Check sheet for the modelled part. Datum: model origin and axes. Units: mm. A direction names the side the tool comes from. Give positions to 0.01 mm unless a question says otherwise; leave off trailing zeros. Loops run counter-clockwise (first coordinate to the right, second up) from the corner with the lowest first, then second, coordinate; pieces in that order, holes last. Notation, with made-up numbers: M 85.25,56 L 121.25,56 A18 ccw 121.25,90 Z; hole C 58.5,63 d11. An arc over 180 degrees is marked long. Write each question's results on one line, items separated by ' | '. Start each with the question number.
1. Sectioned sample at A-A on y = 0.75. Record the cut outline in (x, z), and give its area (3 significant figures).
2. Material ranges on line 1 along Z through (x, y) = (-1.5, 0.5); line 2 along X through (y, z) = (2.75, -0.75); line 3 along X through (y, z) = (1.75, -1.25), recorded low to high.
3. Draft check along X on faces 4 (the conical face through (-2.065, 4.936, -3.597)), 5 (the cylindrical face through (0.631, 4.892, -2.003)), 6 (the conical face through (2.083, 4.936, -3.587)). Enter one of: pulls with the +X half, pulls with the -X half, needs draft (parallel to the pull), parting line crosses it, or undercut.
4. Go/stop test with flat-tipped pins: pin 1 (2 mm diameter, centred on y = 3, z = 2.5, fed in from +X); pin 2 (4 mm diameter, centred on x = 0, z = 0, fed in from -Y); pin 3 (3 mm diameter, centred on y = 5.5, z = -2.5, fed in from +X); pin 4 (1 mm diameter, centred on y = 3.5, z = 3, fed in from -X). Record where each tip stops, or that it passes through.
5. Tool access check on faces 1 (the cylindrical face through (-0.1, 2, 2.5)), 2 (the conical face through (-4.15, 0.087, -0.01)), 3 (the cylindrical face through (3.905, 5.416, 0.867)). Record the directions out of +Z, -Z, +X, -X, +Y, -Y that give a thin tool (end or side, any length) a straight path to the whole face; none if there is none.
```python
from build123d import *

# Parameters (mm, degrees)
ESQUISSE2_OUTSIDE_W     = 16.754
ESQUISSE2_OUTSIDE_H     = 16.754
ENL_V_MAT_EXTRU_2_DEPTH = 7.3000001


with BuildPart() as part:
    # Esquisse1 → Base-Révolution (revolve)
    with BuildSketch(Plane.XY, mode=Mode.PRIVATE) as base_r_volution_sk:
        with BuildLine():
            Line((3, 5.800000004), (3.499999996, 5.800000004))
            Line((3.499999996, 5.800000004), (3.499999996, 4.33246532))
            Line((3.499999996, 4.33246532), (2.5, 4.064516129))
            Line((2.5, 4.064516129), (2.5, 0))
            Line((2.5, 0), (4, 0))
            Line((4, 0), (5.656854249, 0.956585264))
            Line((5.656854249, 0.956585264), (5.656854249, 4.064516129))
            Line((5.656854249, 4.064516129), (3.999999993, 5.02110138))
            Line((3.999999993, 5.02110138), (3.999999993, 5.800000004))
            ThreePointArc((3.999999993, 5.800000004), (3.499999996, 6.3), (3, 5.800000004))
        make_face()
    revolve(base_r_volution_sk.sketch.rotate(Axis((0, 0, 0), (0, 1, 0)), 90), axis=Axis((0, 0, 0), (0, 1, 0)))  # turned: the seam where the file's is

    # Esquisse2 outside → Enlèv. mat.-Extru.2 (cut, through all)
    with BuildSketch(Plane(origin=(0, 0, 0), x_dir=(1, 0, 0), z_dir=(0, 1, 0))):
        Rectangle(ESQUISSE2_OUTSIDE_W, ESQUISSE2_OUTSIDE_H)
        Polygon((-2.309401077, 4), (2.309401077, 4), (4.618802154, 0), (2.309401077, -4), (-2.309401077, -4), (-4.618802154, 0), align=None, mode=Mode.SUBTRACT)
    extrude(amount=ENL_V_MAT_EXTRU_2_DEPTH, mode=Mode.SUBTRACT)

    # Esquisse4 → Boss.-Révol.1 (revolve)
    with BuildSketch(Plane.XY, mode=Mode.PRIVATE) as boss_r_vol_1_sk:
        Polygon((2.1, 3.957336452), (2.1, 5.800000004), (3.499999996, 5.800000004), (3.499999996, 4.33246532), align=None)
    revolve(boss_r_vol_1_sk.sketch.rotate(Axis((0, 5.02110138, 0), (0, -1, 0)), 270), axis=Axis((0, 5.02110138, 0), (0, -1, 0)))  # turned: the seam where the file's is


solid = part.part
```
Output values:
1) outline: M -4.62,0 L -2.31,-4 L 2.31,-4 L 4.62,0 L 2.31,4 L -2.31,4 Z; hole C 0,0 d5 | area: 35.8 mm2
2) line 1: -4 to -2, 2 to 4 | line 2: -4.19 to -2.38, 2.38 to 4.19 | line 3: -3.9 to -2.17, 2.17 to 3.9
3) face 4: pulls with the -X half | face 5: undercut | face 6: pulls with the +X half
4) pin 1: x = 3.75 | pin 2: through | pin 3: x = 3.98 | pin 4: x = -3.18
5) face 1: -Y | face 2: -X, -Y | face 3: +Y
